Print and shaded views of the part. All mm, measured from the part's lowest x, y and z. A direction names the side the tool comes from. Coordinates: 2 decimals unless noted, no trailing zeros. Order: outer loops, then holes, each group sorted by start corner. A loop starts at its lowest first (then second) coordinate and runs counter-clockwise, first axis right, second up.
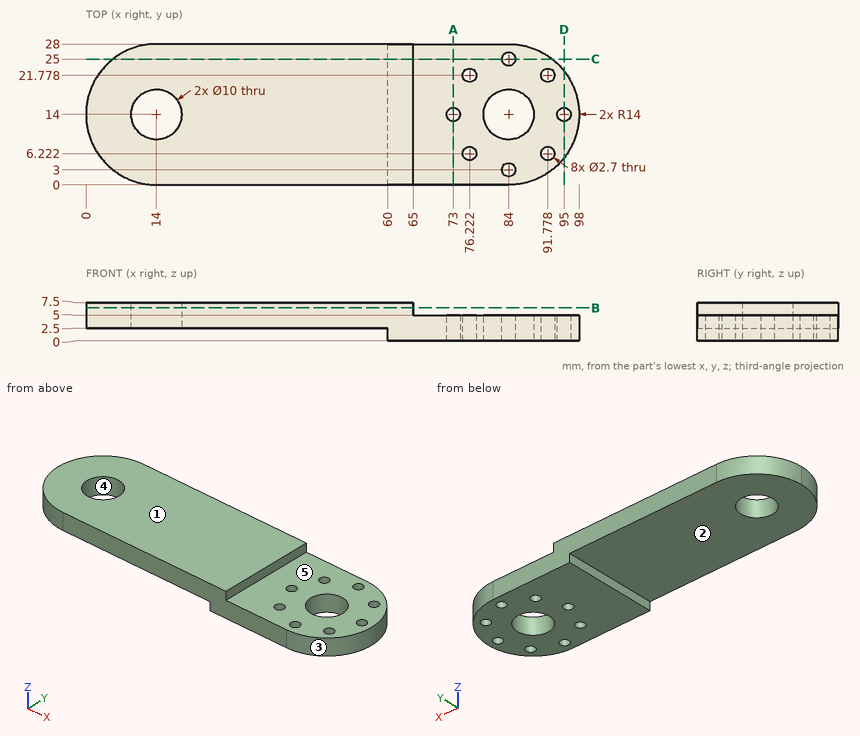
Q1. Cut at B-B, the plane z = 6.5. List the corners of the cut face in (x, y), plus the area to 3 significant figures.
Established:
outline: (14, 0) - (65, 0) - (65, 28) - (14, 28) arc R14 ccw to start; hole circle Ø10 at (14, 14)
area: 1,660 mm2
Q2. Mould opens along X. For the marked faces 3, 4 and 5 say: pulls with the +X half, pulls with the -X half, needs draft (parallel to the pull), parting line crosses it, or undercut.
Established:
face 3: pulls with the +X half
face 4: undercut
face 5: needs draft
Q3. Cut at C-C, the plane y = 25. List the corners of the cut face in (x, z).
Established:
outline: (5.34, 2.5) - (60, 2.5) - (60, 0) - (82.65, 0) - (82.65, 5) - (65, 5) - (65, 7.5) - (5.34, 7.5) - close; (85.35, 0) - (92.66, 0) - (92.66, 5) - (85.35, 5) - close
Q4. Cut at A-A, the plane x = 73. List the corners of the cut face in (y, z).
Established:
outline: (0, 0) - (12.65, 0) - (12.65, 5) - (0, 5) - close; (15.35, 0) - (28, 0) - (28, 5) - (15.35, 5) - close
Q5. Probe line 1 (X direction, y = 23, z = 1) (1 decimal); line 2 (X direction, y = 17, z = 4.5) (1 decimal); line 3 (Z direction, x = 42, y = 23.5). List the from-to ranges inside material, lowest first.
Established:
line 1: x = 60 to 75.6, 76.8 to 91.2, 92.4 to 94.7
line 2: x = 0.3 to 10, 18 to 80, 88 to 97.7
line 3: z = 2.5 to 7.5
Q6. Which spindle directions (+Z, -Z, +X, -X, +Y, -Y) get a long thin tool onto all of the face, cutting with end or side? Do the marked faces 1 and 2. Say none if no direction does.
Established:
face 1: +Z, +X, -X, +Y, -Y
face 2: -Z, -X, +Y, -Y
Q7. Cut at D-D, the plane x = 95. List the corners of the cut face in (y, z), plus the area to 3 significant figures.
Established:
outline: (5.34, 0) - (12.65, 0) - (12.65, 5) - (5.34, 5) - close; (15.35, 0) - (22.66, 0) - (22.66, 5) - (15.35, 5) - close
area: 73.1 mm2
Q8. Drop flat-ended pins along their axis: P1, Ø1.5, axis at y = 9, z = 2.5, coming from the -X side; P2, Ø2, axis at x = 76.22, y = 6.22, coming from the -Z side; P3, Ø2, axis at y = 19, z = 6.5, coming from the +X side; P4, Ø3, axis at x = 60, y = 14.5, coming from the -Z side. Give the stop position or say it passes through.
Established:
P1: stops at x = 0.66
P2: passes through
P3: stops at x = 65
P4: stops at z = 0
